from build123d import *

# Parameters (mm, degrees)
F1_DEPTH = 3.175
F0_W     = 36.8901663726
F0_H     = 9.525
F2_DEPTH = 3.175


with BuildPart() as f1:
    # F0 (on Top) → F1 (new body)
    with BuildSketch(Plane.XY):
        with BuildLine():
            Line((-18.4450831863, 4.7625), (18.4450831863, 4.7625))
            ThreePointArc((18.4450831863, 4.7625), (0, 19.05), (-18.4450831863, 4.7625))
        make_face()
    extrude(amount=F1_DEPTH)



with BuildPart() as f1b:
    # F0 (on Top) → F1, piece 2 (new body)
    with BuildSketch(Plane.XY):
        with BuildLine():
            ThreePointArc((-18.4450831863, -4.7625), (0, -19.05), (18.4450831863, -4.7625))
            Line((18.4450831863, -4.7625), (-18.4450831863, -4.7625))
        make_face()
    extrude(amount=F1_DEPTH)


with BuildPart() as f1_1:
    add(f1.part)

    add(f1b.part)  # F2 merges F1b
    # F0 (on Top) → F2 (join)
    with BuildSketch(Plane.XY):
        with BuildLine():
            ThreePointArc((18.4450831863, -4.7625), (18.8981657139, -2.4003817718), (19.05, 0))
            ThreePointArc((19.05, 0), (18.8981657139, 2.4003817718), (18.4450831863, 4.7625))
            Line((18.4450831863, 4.7625), (18.4450831863, -4.7625))
        make_face()
        with BuildLine():
            Line((-18.4450831863, 4.7625), (18.4450831863, 4.7625))
            ThreePointArc((18.4450831863, 4.7625), (0, 19.05), (-18.4450831863, 4.7625))
        make_face()
        Rectangle(F0_W, F0_H)
        with BuildLine():
            ThreePointArc((-18.4450831863, -4.7625), (0, -19.05), (18.4450831863, -4.7625))
            Line((18.4450831863, -4.7625), (-18.4450831863, -4.7625))
        make_face()
        with BuildLine():
            Line((-18.4450831863, -4.7625), (-18.4450831863, 4.7625))
            ThreePointArc((-18.4450831863, 4.7625), (-19.05, 0), (-18.4450831863, -4.7625))
        make_face()
    extrude(amount=-F2_DEPTH)


solid = f1_1.part
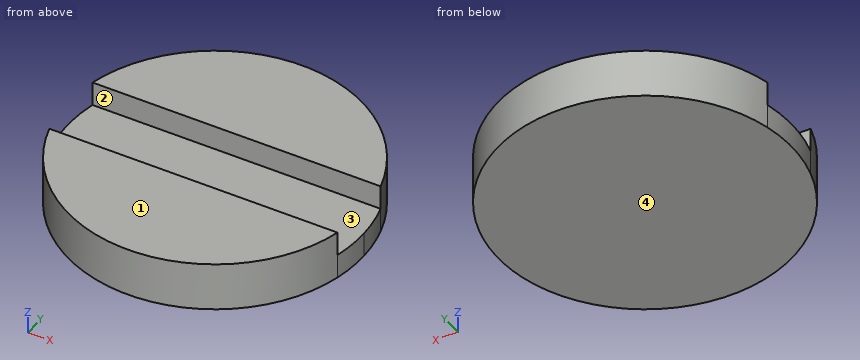
Can you work these out from the model? Positions are in its coordinate system, mm. Face numbers are marked on the shaded views. A direction names the side the tool comes from. Coordinates: 2 decimals unless noted, no trailing zeros. Loops run counter-clockwise (first coordinate to the right, second up) from the corner with the lowest first, then second, coordinate; pieces in that order, holes last. Notation, with made-up numbers: (-29.5, 83) - (18.5, 83) arc R20 cw to (18.5, 99) - close; hole circle Ø1 at (82.5, 51). An arc over 180 degrees is marked (long way). Answer as a JSON object with one key per item and string values. Group by question number.
Item 1: If I drill on L1, parallel to Z at x = 17.5, y = 0.5 (3 decimals); L2, parallel to Y at x = 5.5, z = 2.25; L3, parallel to Y at x = 9.5, z = 0.5, over which ranges is the centre line in solid material (lowest first)? Write a range as from..to.
Item 2: On a 3-axis mill with a long thin cutter (end or side, diameter ignored), from which of +Z, -Z, +X, -X, +Y, -Y can I reach the whole of each face in a straight line? I mean the marked faces 3 and 4. Say none if no direction works.
Item 3: If we section it at A-A (x = 10.5): List the corners of the cut face in (y, z) for me (1 decimal).
Item 4: For pin 1 (3.5 mm diameter, centred on x = 8, z = 1.5, fed in from -Y); pin 2 (2 mm diameter, centred on x = -15, z = -2.5, fed in from +Y); pin 3 (3 mm diameter, centred on x = -7.5, y = -0.5, fed in from +Z), each with a flat end and sliding along its axis, tell me the tip position at first contact or that it passes through.
Item 5: If we section it at D-D (y = -5.5): List the corners of the cut face in (x, z) for me (3 decimals), plus the area to 3 significant figures.
Item 6: If we section it at C-C (z = -0.75): List the corners of the cut face in (x, y) for me.
Item 7: If we section it at B-B (z = 2.5): List the corners of the cut face in (x, y) for me, plus the area to 3 significant figures.
Item 8: If we mould it in two halves opening along Y, with no side actions, what happens to the marked faces 1 and 2? For each: released by +Y, released by -Y, zero draft, split by the parting line, or undercut.
Returned:
{
 "1": {"L1": "z = -3.175..0", "L2": "y = -18.24..-4.76, 4.76..18.24", "L3": "y = -16.51..-4.76, 4.76..16.51"},
 "2": {"face 3": "+Z, +X, -X", "face 4": "-Z, +X, -X, +Y, -Y"},
 "3": {"outline": "(-15.9, -3.2) - (15.9, -3.2) - (15.9, 3.2) - (4.8, 3.2) - (4.8, 0) - (-4.8, 0) - (-4.8, 3.2) - (-15.9, 3.2) - close"},
 "4": {"pin 1": "stops at y = -18", "pin 2": "stops at y = 12.92", "pin 3": "stops at z = 0"},
 "5": {"outline": "(-18.239, -3.175) - (18.239, -3.175) - (18.239, 3.175) - (-18.239, 3.175) - close", "area": "232 mm²"},
 "6": {"outline": "circle Ø38.1 at (0, 0)"},
 "7": {"outline": "(-18.45, -4.76) arc R19.05 ccw to (18.45, -4.76) - close; (-18.45, 4.76) - (18.45, 4.76) arc R19.05 ccw to start", "area": "781 mm²"},
 "8": {"face 1": "zero draft", "face 2": "undercut"}
}
